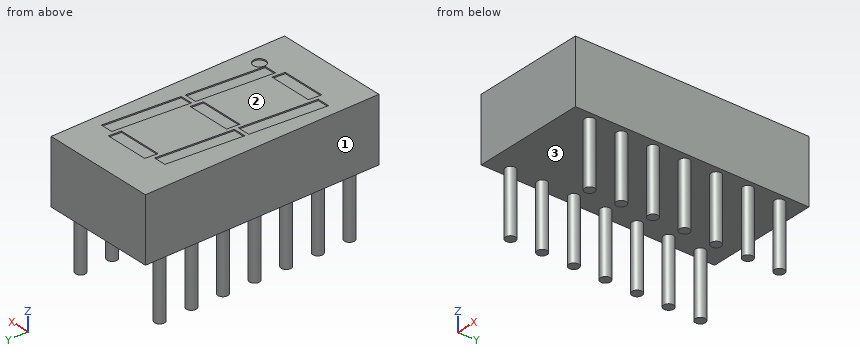
```python
from build123d import *

# Parameters (mm, degrees)
SKETCH1_W           = 9.08
SKETCH1_H           = 18.75
BODY_DEPTH          = 5.08
SKETCH2_R           = 0.4
PINS_DEPTH          = 5
PIN_PATTERN_1_COUNT = 4
PIN_PATTERN_1_PITCH = 2.54
PIN_PATTERN_2_COUNT = 4
PIN_PATTERN_2_PITCH = 2.54
SKETCH3_R           = 0.5
LED_DISPLAY_DEPTH   = 0.1


with BuildPart() as part:
    # Sketch1 → Body (new body)
    with BuildSketch(Plane.XY):
        Rectangle(SKETCH1_W, SKETCH1_H)
    extrude(amount=BODY_DEPTH)

    # Sketch2 → Pins (add)
    with BuildSketch(Plane(origin=(0, 0, 0), x_dir=(-1, 0, 0), z_dir=(0, 0, -1))):
        with Locations((-3.81, 0)):
            Circle(SKETCH2_R)
        with Locations((3.81, 0)):
            Circle(SKETCH2_R)
    pins = extrude(amount=PINS_DEPTH)

    # Pin Pattern 1: Pins ×4
    with Locations(*[(0, -i * PIN_PATTERN_1_PITCH, 0) for i in range(1, PIN_PATTERN_1_COUNT)]):
        add(pins)

    # Pin Pattern 2: Pins ×4
    with Locations(*[(0, i * PIN_PATTERN_2_PITCH, 0) for i in range(1, PIN_PATTERN_2_COUNT)]):
        add(pins)

    # Sketch3 → LED Display (cut)
    with BuildSketch(Plane.XY.offset(5.08)):
        with Locations((3.074773804, -6.127168189)):
            Circle(SKETCH3_R)
        Polygon((-1.521772911, 6.127168189), (-2.044707367, 0.15), (-3.048527205, 0.15), (-2.525592748, 6.127168189), align=None)
        Polygon((-3.597708261, -6.127168189), (-2.593888423, -6.127168189), (-2.070953966, -0.15), (-3.074773804, -0.15), align=None)
        Polygon((2.593888423, 6.127168189), (2.070953966, 0.15), (3.074773804, 0.15), (3.597708261, 6.127168189), align=None)
        Polygon((1.521772911, -6.127168189), (2.525592748, -6.127168189), (3.048527205, -0.15), (2.044707367, -0.15), align=None)
        Polygon((-1.712940384, 0.5), (-1.800429047, -0.5), (1.712940384, -0.5), (1.800429047, 0.5), align=None)
        Polygon((-1.264371291, 5.627168189), (-1.176882628, 6.627168189), (2.336486803, 6.627168189), (2.24899814, 5.627168189), align=None)
        Polygon((-2.24899814, -5.627168189), (-2.336486803, -6.627168189), (1.176882628, -6.627168189), (1.264371291, -5.627168189), align=None)
    extrude(amount=-LED_DISPLAY_DEPTH, mode=Mode.SUBTRACT)


solid = part.part
```
Could you check a few things on this model? Use its own coordinates, in mm. Face numbers are marked on the shaded views. Give positions to 0.01 mm unless a question says otherwise; leave off trailing zeros. Loops run counter-clockwise (first coordinate to the right, second up) from the corner with the lowest first, then second, coordinate; pieces in that order, holes last. Notation, with made-up numbers: (-10.5, 87.5) - (1.5, 87.5) arc R18 ccw to (1.5, 99.5) - close; hole circle Ø3 at (72.25, -8.5). An arc over 180 degrees is marked (long way). Use one line per item in the form item = value.
1. Thinking about a two-plate mould opening in X: for the marked faces 1, 2 and 3, which applies, released by +X, released by -X, zero draft, split by the parting line, or undercut?
Response values:
face_1 = released by -X
face_2 = zero draft
face_3 = undercut
2. I want a section at D-D (y = -5.08). Please give me the cut outline in (x, z).
Response values:
outline = (-4.54, 0) - (-4.21, 0) - (-4.21, -5) - (-3.41, -5) - (-3.41, 0) - (3.41, 0) - (3.41, -5) - (4.21, -5) - (4.21, 0) - (4.54, 0) - (4.54, 5.08) - (2.62, 5.08) - (2.62, 4.98) - (1.61, 4.98) - (1.61, 5.08) - (-2.5, 5.08) - (-2.5, 4.98) - (-3.51, 4.98) - (-3.51, 5.08) - (-4.54, 5.08) - close
3. I need wall thicknesses on probe 1 along Z at (x, y) = (0.75, 4.5); probe 2 along Z at (x, y) = (-2.5, -0.5); probe 3 along X at (y, z) = (-5, -3). Which ranges of each line are inside material? Lowest first, please.
Response values:
probe_1 = 0 to 5.08
probe_2 = 0 to 4.98
probe_3 = -4.2 to -3.42, 3.42 to 4.2
4. I'm going to push a flat-ended pin straight in: pin 1 Ø0.8 at (x, y) = (3, -6) entering from +Z. Where does the tip first touch, or does it pass through?
Response values:
pin_1 = 5.08
5. I want a section at C-C (y = -7.62). Please give me the cut outline in (x, z).
Response values:
outline = (-4.54, 0) - (-4.21, 0) - (-4.21, -5) - (-3.41, -5) - (-3.41, 0) - (3.41, 0) - (3.41, -5) - (4.21, -5) - (4.21, 0) - (4.54, 0) - (4.54, 5.08) - (-4.54, 5.08) - close
6. I want a section at A-A (z = -1.75). Give the number of separate pieces and of enclosed holes in the cut face, and give its area (3 significant figures).
Response values:
separate_pieces = 14
enclosed_holes = 0
area = 7.04 mm²
